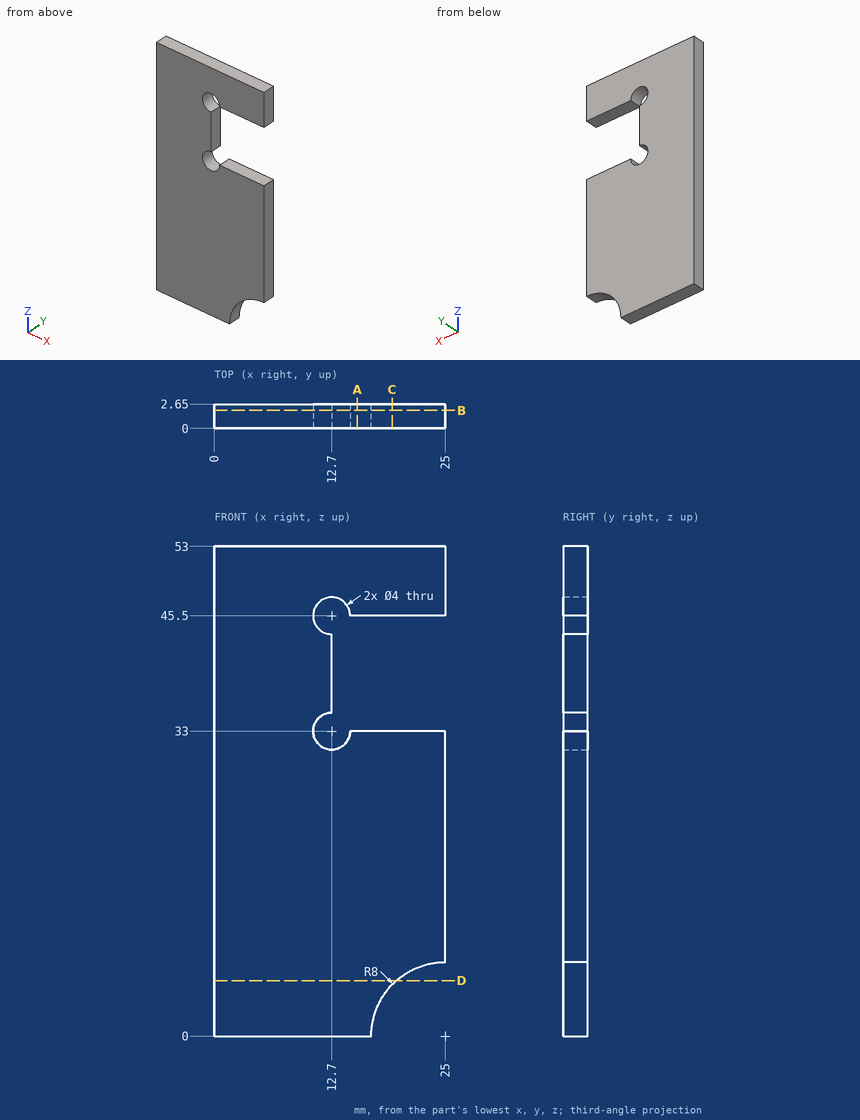
Geometry: see drawing. Coordinates: mm, zero at the bounding-box minimum. Coordinates: 2 decimals unless noted, no trailing zeros. Order: outer loops, then holes, each group sorted by start corner. A loop starts at its lowest first (then second) coordinate and runs counter-clockwise, first axis right, second up. Notation, with made-up numbers: M -27.75,78.5 L 24.25,78.5 A34 ccw 24.25,111.5 Z; hole C -25.75,70.25 d10. An arc over 180 degrees is marked long. Write item = value, one per line. Start each with the question number.
(1) Section D-D on z = 6. Output: boundary loops of the cut face in (x, y), and give its area (3 significant figures).
(2) First-contact query: P1, Ø0.8, axis at x = 18.5, y = 2, coming from the -Z side; P2, Ø3, axis at x = 12.7, z = 33, coming from the -Y side; P3, Ø1, axis at x = 22.5, y = 1.5, coming from the -Z side. Flat tips, straight axial feed; report the tip coordinate or a pass-through.
(3) Section B-B on y = 1.95. Output: boundary loops of the cut face in (x, z), and give its area (3 significant figures).
(4) Section A-A on x = 15.5. Output: boundary loops of the cut face in (y, z), and give its area (3 significant figures).
(5) Section C-C on x = 19.25. Output: boundary loops of the cut face in (y, z), and give its area (3 significant figures).
(6) Line query: line 1 along Z through (x, y) = (23, 0.2); line 2 along Z through (x, y) = (20.75, 0.95); line 3 along X through (y, z) = (2.3, 45). Output: solid intervals per line, ascending. Write a range as [from, to].
Result set:
q1.outline = M 0,0 L 19.71,0 L 19.71,2.65 L 0,2.65 Z
q1.area = 52.2 mm²
q2.P1 = 4.05
q2.P2 = through
q2.P3 = 7.42
q3.outline = M 0,0 L 17,0 A8 cw 25,8 L 25,33 L 14.7,33 A2 cw long 12.7,35 L 12.7,43.5 A2 cw long 14.7,45.5 L 25,45.5 L 25,53 L 0,53 Z
q3.area = 1,100 mm²
q4.outline = M 0,0 L 2.65,0 L 2.65,33 L 0,33 Z; M 0,45.5 L 2.65,45.5 L 2.65,53 L 0,53 Z
q4.area = 107 mm²
q5.outline = M 0,5.56 L 2.65,5.56 L 2.65,33 L 0,33 Z; M 0,45.5 L 2.65,45.5 L 2.65,53 L 0,53 Z
q5.area = 92.6 mm²
q6.line_1 = [7.75, 33], [45.5, 53]
q6.line_2 = [6.78, 33], [45.5, 53]
q6.line_3 = [0, 10.76]
